```python
from build123d import *

# Parameters (mm, degrees)
F0_R     = 63.5
F0_W     = 37
F0_H     = 37
F0_R_2   = 10
F1_DEPTH = 5


with BuildPart() as f1:
    # F0 (on Top) → F1 (new body)
    with BuildSketch(Plane.XY):
        Circle(F0_R)
        with Locations((-31.75, 0)):
            Rectangle(F0_W, F0_H, mode=Mode.SUBTRACT)
        Circle(F0_R_2, mode=Mode.SUBTRACT)
        with Locations((31.75, 0)):
            Rectangle(F0_W, F0_H, mode=Mode.SUBTRACT)
    extrude(amount=F1_DEPTH)


solid = f1.part
```
Can you work these out from the model? Positions are in its coordinate system, mm. A direction names the side the tool comes from. Round coordinates to 2 decimals unless told otherwise and drop trailing zeros. Order: outer loops, then holes, each group sorted by start corner. A loop starts at its lowest first (then second) coordinate and runs counter-clockwise, first axis right, second up.
(1) On a 3-axis mill with a long thin cutter (end or side, diameter ignored), from which of +Z, -Z, +X, -X, +Y, -Y can I reach the whole of each face in a straight line? I mean faces 1 (the face through (50.25, 0, 2)), 2 (the face through (13, 1, 5)). Say none if no direction works.
Results are:
face 1: +Z, -Z
face 2: +Z, +X, -X, +Y, -Y
(2) We'd pull the mould along X, two halves only. Please class faces 3 (the face through (13, 1, 0)), 4 (the face through (-32, -18.5, 2)), 5 (the face through (-13.77, -61.99, 2.46)): +X half, -X half, draft (parallel to the pull), parting line (faces both ways), or undercut.
Results are:
face 3: draft
face 4: undercut
face 5: parting line
(3) I'm going to push flat-ended pins straight in: pin 1 (1.5 mm diameter, centred on x = 33.5, z = 1.5, fed in from -Y); pin 2 (2 mm diameter, centred on x = 31.5, z = 4.5, fed in from +Y); pin 3 (1.5 mm diameter, centred on x = -40, z = 2, fed in from -Y). Where does each tip first touch, or does it pass through?
Results are:
pin 1: stops at y = -54.4
pin 2: stops at y = 55.7
pin 3: stops at y = -49.92
(4) If I drill on L1, parallel to X at y = -12, z = 3.8; L2, parallel to Y at x = 0, z = 2.9; L3, parallel to X at y = 16, z = 1.8, over which ranges is the centre line in solid material (lowest first)?
Results are:
L1: x = -62.36 to -50.25, -13.25 to 13.25, 50.25 to 62.36
L2: y = -63.5 to -10, 10 to 63.5
L3: x = -61.45 to -50.25, -13.25 to 13.25, 50.25 to 61.45
(5) If we section it at A-A (x = 0): Please give me the cut outline in (y, z), plus the area to 3 significant figures.
Results are:
outline: (-63.5, 0) - (-10, 0) - (-10, 5) - (-63.5, 5) - close; (10, 0) - (63.5, 0) - (63.5, 5) - (10, 5) - close
area: 535 mm2
(6) If we section it at B-B (y = 0): Please give me the cut outline in (x, z).
Results are:
outline: (-63.5, 0) - (-50.25, 0) - (-50.25, 5) - (-63.5, 5) - close; (-13.25, 0) - (-10, 0) - (-10, 5) - (-13.25, 5) - close; (10, 0) - (13.25, 0) - (13.25, 5) - (10, 5) - close; (50.25, 0) - (63.5, 0) - (63.5, 5) - (50.25, 5) - close
(7) If we section it at D-D (x = 33.5): Please give me the cut outline in (y, z).
Results are:
outline: (-53.94, 0) - (-18.5, 0) - (-18.5, 5) - (-53.94, 5) - close; (18.5, 0) - (53.94, 0) - (53.94, 5) - (18.5, 5) - close
(8) If we section it at C-C (z = 2.9): Please give me the cut outline in (x, y).
Results are:
outline: circle Ø127 at (0, 0); hole (-50.25, -18.5) - (-13.25, -18.5) - (-13.25, 18.5) - (-50.25, 18.5) - close; hole circle Ø20 at (0, 0); hole (13.25, -18.5) - (50.25, -18.5) - (50.25, 18.5) - (13.25, 18.5) - close
